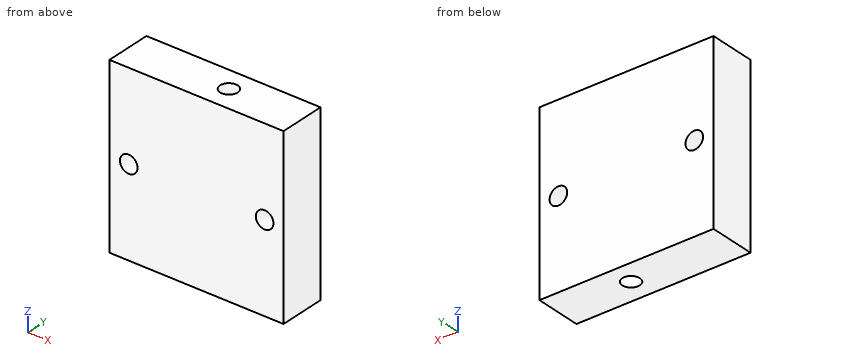
from build123d import *

# Parameters (mm, degrees)
SKETCH2_W        = 495
SKETCH2_H        = 500
HIPS_DEPTH       = 132
SKETCH3_R        = 25
FEMUR_HOLE_DEPTH = 574.306418942
SKETCH4_R        = 25
TAIL_HOLE_DEPTH  = 376.739603981
SKETCH5_R        = 25
NECK_HOLE_DEPTH  = 376.739603981


with BuildPart() as part:
    # Sketch2 → Hips (new body)
    with BuildSketch(Plane(origin=(0, 0, 0), x_dir=(1, 0, 0), z_dir=(0, 1, 0))):
        Rectangle(SKETCH2_W, SKETCH2_H)
    extrude(amount=HIPS_DEPTH)

    # Sketch3 → Femur-hole (cut, through all)
    with BuildSketch(Plane.XY.offset(250)):
        with Locations((38.58686963, 67.285203145)):
            Circle(SKETCH3_R)
    extrude(amount=-FEMUR_HOLE_DEPTH, mode=Mode.SUBTRACT)

    # Sketch4 → Tail-hole (cut, through all)
    with BuildSketch(Plane.XZ):
        with Locations(Location((193.717960243, 0, 0), (0, 0, 270))):
            Circle(SKETCH4_R)
    extrude(amount=-TAIL_HOLE_DEPTH, mode=Mode.SUBTRACT)

    # Sketch5 → Neck-hole (cut, through all)
    with BuildSketch(Plane.XZ):
        with Locations(Location((-192.698108673, 0, 0), (0, 0, 270))):
            Circle(SKETCH5_R)
    extrude(amount=-NECK_HOLE_DEPTH, mode=Mode.SUBTRACT)


solid = part.part
Design review of the part built by this model. Coordinates are the model's own, in mm. Give positions to 0.01 mm unless a question says otherwise; leave off trailing zeros. Loops run counter-clockwise (first coordinate to the right, second up) from the corner with the lowest first, then second, coordinate; pieces in that order, holes last. Notation, with made-up numbers: (34.25, -18) - (78.25, -18) arc R21 cw to (78.25, 2) - close; hole circle Ø2 at (83, 55.5). An arc over 180 degrees is marked (long way). Use CSV: the item, a comma, the result in double quotes. Start each with the question number.
1. Add section C-C (x = 24.5). State the section outline as (y, z) points, plus the area to 3 significant figures.
2. Add section B-B (z = 0). State the section outline as (x, y) points, plus the area to 3 significant figures.
3. Wall thickness on L1, parallel to X at y = 101, z = 0; L2, parallel to Z at x = -192, y = 96.5; L3, parallel to X at y = 52, z = -124: over which ranges is each line inside the solid? List them lowest first.
4. Add section D-D (z = 135.5). State the section outline as (x, y) points, plus the area to 3 significant figures.
5. Add section A-A (y = 84). State the section outline as (x, z) points, plus the area to 3 significant figures.
Results found:
1,outline,"(0, -250) - (46.63, -250) - (46.63, 250) - (0, 250) - close; (87.94, -250) - (132, -250) - (132, 250) - (87.94, 250) - close"
1,area,"45,300 mm²"
2,outline,"(-247.5, 0) - (-217.7, 0) - (-217.7, 132) - (-247.5, 132) - close; (-167.7, 0) - (168.72, 0) - (168.72, 132) - (-167.7, 132) - close; (218.72, 0) - (247.5, 0) - (247.5, 132) - (218.72, 132) - close; hole circle Ø50 at (38.59, 67.29)"
2,area,"50,200 mm²"
3,L1,"x = -247.5 to -217.7, -167.7 to 168.72, 218.72 to 247.5"
3,L2,"z = -250 to -24.99, 24.99 to 250"
3,L3,"x = -247.5 to 18.8, 58.37 to 247.5"
4,outline,"(-247.5, 0) - (247.5, 0) - (247.5, 132) - (-247.5, 132) - close; hole circle Ø50 at (38.59, 67.29)"
4,area,"63,400 mm²"
5,outline,"(-247.5, -250) - (20, -250) - (20, 250) - (-247.5, 250) - close; (57.18, -250) - (247.5, -250) - (247.5, 250) - (57.18, 250) - close; hole circle Ø50 at (-192.7, 0); hole circle Ø50 at (193.72, 0)"
5,area,"225,000 mm²"
